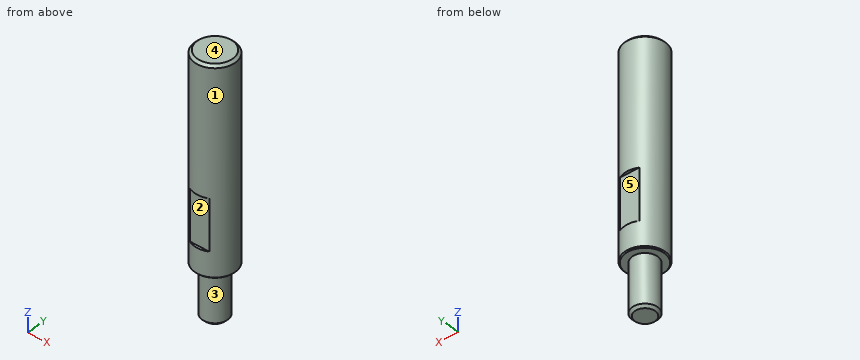
from build123d import *

# Parameters (mm, degrees)
SKETCH_1_R          = 4
EXTRUDE_1_DEPTH     = 25
CUT_EXTRUDE_START   = -10
SKETCH_2_R          = 4
SKETCH_2_R_2        = 2.5
CUT_EXTRUDE_1_DEPTH = 10
CHAMFER_1_SIZE      = 0.5
CHAMFER_2_SIZE      = 0.2
SKETCH_3_W          = 10
SKETCH_3_H          = 0.502777741
SKETCH_3_H_2        = 0.50277774
CUT_EXTRUDE_2_DEPTH = 5
CHAMFER_3_SIZE      = 0.5


with BuildPart() as part:
    # 草圖1 → 填料-伸長1 (new, symmetric)
    with BuildSketch(Plane.XY):
        Circle(SKETCH_1_R)
    extrude(amount=EXTRUDE_1_DEPTH, both=True)

    # 草圖2 → 除料-伸長1 (cut)
    with BuildSketch(Plane(origin=(0, 0, -25), x_dir=(-1, 0, 0), z_dir=(0, 0, -1)).offset(CUT_EXTRUDE_START)):
        Circle(SKETCH_2_R)
        Circle(SKETCH_2_R_2, mode=Mode.SUBTRACT)
    extrude(amount=CUT_EXTRUDE_1_DEPTH, mode=Mode.SUBTRACT)

    # 導角1
    chamfer_1_edges = [part.edges().sort_by_distance(p)[0] for p in [
        (2.5, 0, -25),
    ]]
    chamfer(chamfer_1_edges, length=CHAMFER_1_SIZE)

    # 導角2
    chamfer_2_edges = [part.edges().sort_by_distance(p)[0] for p in [
        (-4, 0, -15),
    ]]
    chamfer(chamfer_2_edges, length=CHAMFER_2_SIZE)

    # 草圖3 → 除料-伸長2 (cut, symmetric)
    with BuildSketch(Plane(origin=(0, 0, 0), x_dir=(0, 0, -1), z_dir=(1, 0, 0))):
        with Locations((5, 3.754166611)):
            Rectangle(SKETCH_3_W, SKETCH_3_H)
        with Locations((5, -3.74861113)):
            Rectangle(SKETCH_3_W, SKETCH_3_H_2)
    extrude(amount=CUT_EXTRUDE_2_DEPTH, both=True, mode=Mode.SUBTRACT)

    # 導角3
    chamfer_3_edges = [part.edges().sort_by_distance(p)[0] for p in [
        (-4, 0, 25),
    ]]
    chamfer(chamfer_3_edges, length=CHAMFER_3_SIZE)


solid = part.part
The listing builds one solid part. Answer for the finished solid, in the listing's coordinates (mm). Face numbers are marked on the shaded views. A direction names the side the tool comes from. Give positions to 0.01 mm unless a question says otherwise; leave off trailing zeros. Write each loop counter-clockwise with the first axis right and the second up, starting at its lowest first coordinate (ties: lowest second). Pieces come first, ordered by that corner, then holes. Notation, with made-up numbers: (-8, -25.5) -> (31, -25.5) arc R15 ccw to (31, -15.5) -> close; hole circle Ø1 at (-34.75, -11). An arc over 180 degrees is marked (long way). Use a Markdown table: item, result.
(1) Section C-C, the plane z = -14 is taken. Determine the outline of the cut face in (x, y).
Return value:
| item | result |
|---|---|
| outline | circle Ø8 at (0, 0) |
(2) Section A-A, the plane y = 0 is taken. Determine the outline of the cut face in (x, z).
Return value:
| item | result |
|---|---|
| outline | (-4, -14.8) -> (-3.8, -15) -> (-2.5, -15) -> (-2.5, -24.5) -> (-2, -25) -> (2, -25) -> (2.5, -24.5) -> (2.5, -15) -> (3.8, -15) -> (4, -14.8) -> (4, 24.5) -> (3.5, 25) -> (-3.5, 25) -> (-4, 24.5) -> close |
(3) Section B-B, the plane x = 0 is taken. Determine the outline of the cut face in (y, z).
Return value:
| item | result |
|---|---|
| outline | (-4, -14.8) -> (-3.8, -15) -> (-2.5, -15) -> (-2.5, -24.5) -> (-2, -25) -> (2, -25) -> (2.5, -24.5) -> (2.5, -15) -> (3.8, -15) -> (4, -14.8) -> (4, -10) -> (3.5, -10) -> (3.5, 0) -> (4, 0) -> (4, 24.5) -> (3.5, 25) -> (-3.5, 25) -> (-4, 24.5) -> (-4, 0) -> (-3.5, 0) -> (-3.5, -10) -> (-4, -10) -> close |
(4) Determine the mould class of the marked faces 3, 4 and 5 for opening direction Z: released by +Z, released by -Z, zero draft, split by the parting line, or undercut.
Return value:
| item | result |
|---|---|
| face 3 | zero draft |
| face 4 | released by +Z |
| face 5 | undercut |
(5) Section D-D, the plane z = -2 is taken. Determine the outline of the cut face in (x, y).
Return value:
| item | result |
|---|---|
| outline | (-1.94, -3.5) -> (1.94, -3.5) arc R4 ccw to (1.93, 3.5) -> (-1.93, 3.5) arc R4 ccw to start |
(6) Find the intervals of material crossed by probe 1 along Z at (x, y) = (2.25, 1.75); probe 2 along Y at (x, z) = (3.5, 13); probe 3 along X at (y, z) = (1.25, 0), in increasing order. Write a range as from..to.
Return value:
| item | result |
|---|---|
| probe 1 | -15..25 |
| probe 2 | -1.94..1.94 |
| probe 3 | -3.8..3.8 |
(7) For the marked faces 1 and 2, determine the directions among +Z, -Z, +X, -X, +Y, -Y from which every point of the face is accessible in a straight line to the end or side of a thin tool.
Return value:
| item | result |
|---|---|
| face 1 | +Z, -Z |
| face 2 | +X, -X, -Y |
(8) Flat-ended cylindrical pins translate along their axes: P1, Ø2, axis at x = 2.5, y = -2, coming from the -Z side; P2, Ø1.2, axis at x = -0.5, z = -6.5, coming from the +Y side; P3, Ø3, axis at x = 0.5, z = -4, coming from the -Y side. Find the tip coordinate at first contact, or state that the pin passes through.
Return value:
| item | result |
|---|---|
| P1 | z = -24.8 |
| P2 | y = 3.5 |
| P3 | y = -3.5 |
